Can you work these out from the model? Positions are in its coordinate system, mm. A direction names the side the tool comes from. Coordinates: 2 decimals unless noted, no trailing zeros. Loops run counter-clockwise (first coordinate to the right, second up) from the corner with the lowest first, then second, coordinate; pieces in that order, holes last. Notation, with made-up numbers: (-16.75, -31.5) -> (33.25, -31.5) arc R24 cw to (33.25, -9.5) -> close; hole circle Ø1 at (74.5, 89). An arc over 180 degrees is marked (long way). Put each result on its own line as item: value. Start each with the question number.
Item 1: We'd pull the mould along Y, two halves only. Please class faces 5 (the cylindrical face through (0.621, 21.497, 10.749)), 6 (the cylindrical face through (-5.15, 2.02, 18.59)), 7 (the flat face through (0, 15, 14.8)), 8 (the flat face through (0, 5, 3)): pulls with the +Y half, pulls with the -Y half, needs draft (parallel to the pull), parting line crosses it, or undercut.
Item 2: Will these pins go through, and if not, where does the flat tip stop? P1, Ø8, axis at y = 20.5, z = 2, coming from the +X side; P2, Ø6, axis at x = 2, z = 1, coming from the +Y side; P3, Ø0.6, axis at x = -0.5, y = -1.5, coming from the +Z side; P4, Ø6, axis at x = -2.5, z = 12, coming from the -Y side.
Item 3: If we section it at B-B on z = 13: Please give me the cut outline in (x, y), plus the area to 3 significant figures.
Item 4: For faces 1 (the flat face through (-1, -1, 3)), 2 (the flat face through (4.15, 12, 11)), 3 (the flat face through (0, -1, 2)), 4 (the cylindrical face through (5.15, 1.98, 18.59)), which set-ups out of +Z, -Z, +X, -X, +Y, -Y let a thin tool reach every point of the face, with its end or its side?
Item 5: If we section it at A-A on y = 20: Please give me the cut outline in (x, z), plus the area to 3 significant figures.
Item 6: If we section it at C-C on z = 3.5: Please give me the cut outline in (x, y).
Item 7: Please list where these lines run through material, in increasing order: L1, parallel to Y at x = 0, z = 11; L2, parallel to X at y = 20, z = 10.25; L3, parallel to Z at x = -3, y = 7.75. Write a range as from..to.
Item 8: If we section it at D-D on x = 2.5: Please give me the cut outline in (y, z), plus the area to 3 significant figures.
```python
from build123d import *

# Parameters (mm, degrees)
BOSS_EXTRUDE1_DEPTH      = 4.15
BOSS_EXTRUDE1_DEPTH_BACK = 4.15
BOSS_EXTRUDE2_DEPTH      = 18.1
BOSS_EXTRUDE3_DEPTH      = 1
BOSS_EXTRUDE4_DEPTH      = 1
SKETCH7_W                = 2
SKETCH7_H                = 2
BOSS_EXTRUDE5_DEPTH      = 1
BOSS_EXTRUDE5_DEPTH_BACK = 1


with BuildPart() as part:
    # Sketch1 → Boss-Extrude1 (new body, two sides)
    with BuildSketch(Plane(origin=(0, 0, 0), x_dir=(0, 0, -1), z_dir=(1, 0, 0))) as boss_extrude1_sk:
        with BuildLine():
            Line((-18.1, 5), (-18.1, 0))
            Line((-18.1, 0), (0, 0))
            Line((0, 0), (0, 5))
            Line((0, 5), (-6.5, 5))
            ThreePointArc((-6.5, 5), (-6.712132034, 5.087867966), (-6.8, 5.3))
            Line((-6.8, 5.3), (-6.8, 24.8))
            ThreePointArc((-6.8, 24.8), (-6.858578644, 24.941421356), (-7, 25))
            Line((-7, 25), (-14.6, 25))
            ThreePointArc((-14.6, 25), (-14.741421356, 24.941421356), (-14.8, 24.8))
            Line((-14.8, 24.8), (-14.8, 5.3))
            ThreePointArc((-14.8, 5.3), (-14.887867966, 5.087867966), (-15.1, 5))
            Line((-15.1, 5), (-18.1, 5))
        make_face()
    extrude(amount=BOSS_EXTRUDE1_DEPTH)
    extrude(boss_extrude1_sk.sketch, amount=-BOSS_EXTRUDE1_DEPTH_BACK)

    # Sketch2 → Cut-Revolve1 (revolve, cut)
    with BuildSketch(Plane(origin=(0, 0, 0), x_dir=(0, 0, -1), z_dir=(1, 0, 0))):
        Polygon((-14.8, 20), (-14.8, 22), (-14.421, 21.621), (-7.179, 21.621), (-6.8, 22), (-6.8, 20), align=None)
    revolve(axis=Axis((0, 20, 6.8), (0, 0, 1)), mode=Mode.SUBTRACT)

    # Sketch3 → Cut-Revolve2 (revolve, cut)
    with BuildSketch(Plane(origin=(0, 0, 0), x_dir=(0, 0, -1), z_dir=(1, 0, 0))):
        Polygon((-14.8, 11), (-14.8, 13), (-14.421, 12.621), (-7.179, 12.621), (-6.8, 13), (-6.8, 11), align=None)
    revolve(axis=Axis((0, 11, 6.8), (0, 0, 1)), mode=Mode.SUBTRACT)

    # Sketch4 → Boss-Extrude2 (add)
    with BuildSketch(Plane.XY):
        with BuildLine():
            Line((-4.15, 0.75), (4.15, 0.75))
            ThreePointArc((4.15, 0.75), (5.4, 2), (4.15, 3.25))
            Line((4.15, 3.25), (-4.15, 3.25))
            ThreePointArc((-4.15, 3.25), (-5.4, 2), (-4.15, 0.75))
        make_face()
    extrude(amount=BOSS_EXTRUDE2_DEPTH)

    # Sketch5 → Boss-Extrude3 (add)
    with BuildSketch(Plane.XY):
        with BuildLine():
            Line((-4.15, 0.658359214), (-4.15, 0.2))
            ThreePointArc((-4.15, 0.2), (-4.091421356, 0.058578644), (-3.95, 0))
            Line((-3.95, 0), (3.95, 0))
            ThreePointArc((3.95, 0), (4.091421356, 0.058578644), (4.15, 0.2))
            Line((4.15, 0.2), (4.15, 0.658359214))
            ThreePointArc((4.15, 0.658359214), (4.22928651, 0.897404935), (4.435714286, 1.041685153))
            ThreePointArc((4.435714286, 1.041685153), (5.15, 2), (4.435714286, 2.958314847))
            ThreePointArc((4.435714286, 2.958314847), (4.22928651, 3.102595065), (4.15, 3.341640786))
            Line((4.15, 3.341640786), (4.15, 4.8))
            ThreePointArc((4.15, 4.8), (4.091421356, 4.941421356), (3.95, 5))
            Line((3.95, 5), (-3.95, 5))
            ThreePointArc((-3.95, 5), (-4.091421356, 4.941421356), (-4.15, 4.8))
            Line((-4.15, 4.8), (-4.15, 3.341640786))
            ThreePointArc((-4.15, 3.341640786), (-4.22928651, 3.102595065), (-4.435714286, 2.958314847))
            ThreePointArc((-4.435714286, 2.958314847), (-5.15, 2), (-4.435714286, 1.041685153))
            ThreePointArc((-4.435714286, 1.041685153), (-4.22928651, 0.897404935), (-4.15, 0.658359214))
        make_face()
    extrude(amount=-BOSS_EXTRUDE3_DEPTH)

    # Sketch6 → Boss-Extrude4 (add)
    with BuildSketch(Plane.XY.offset(18.1)):
        with BuildLine():
            Line((-4.15, 0.658359214), (-4.15, 0.2))
            ThreePointArc((-4.15, 0.2), (-4.091421356, 0.058578644), (-3.95, 0))
            Line((-3.95, 0), (3.95, 0))
            ThreePointArc((3.95, 0), (4.091421356, 0.058578644), (4.15, 0.2))
            Line((4.15, 0.2), (4.15, 0.658359214))
            ThreePointArc((4.15, 0.658359214), (4.22928651, 0.897404935), (4.435714286, 1.041685153))
            ThreePointArc((4.435714286, 1.041685153), (5.15, 2), (4.435714286, 2.958314847))
            ThreePointArc((4.435714286, 2.958314847), (4.22928651, 3.102595065), (4.15, 3.341640786))
            Line((4.15, 3.341640786), (4.15, 4.8))
            ThreePointArc((4.15, 4.8), (4.091421356, 4.941421356), (3.95, 5))
            Line((3.95, 5), (-3.95, 5))
            ThreePointArc((-3.95, 5), (-4.091421356, 4.941421356), (-4.15, 4.8))
            Line((-4.15, 4.8), (-4.15, 3.341640786))
            ThreePointArc((-4.15, 3.341640786), (-4.22928651, 3.102595065), (-4.435714286, 2.958314847))
            ThreePointArc((-4.435714286, 2.958314847), (-5.15, 2), (-4.435714286, 1.041685153))
            ThreePointArc((-4.435714286, 1.041685153), (-4.22928651, 0.897404935), (-4.15, 0.658359214))
        make_face()
    extrude(amount=BOSS_EXTRUDE4_DEPTH)

    # Sketch7 → Boss-Extrude5 (add, two sides)
    with BuildSketch(Plane(origin=(0, 0, 0), x_dir=(0, 0, -1), z_dir=(1, 0, 0))) as boss_extrude5_sk:
        with Locations((-3, -1)):
            Rectangle(SKETCH7_W, SKETCH7_H)
    extrude(amount=BOSS_EXTRUDE5_DEPTH)
    extrude(boss_extrude5_sk.sketch, amount=-BOSS_EXTRUDE5_DEPTH_BACK)


solid = part.part
```
Solutions:
1. face 5: undercut
1. face 6: parting line crosses it
1. face 7: needs draft
1. face 8: pulls with the +Y half
2. P1: through
2. P2: y = 5
2. P3: z = 4
2. P4: y = 0
3. outline: (-4.15, 0) -> (4.15, 0) -> (4.15, 0.75) arc R1.25 ccw to (4.15, 3.25) -> (4.15, 25) -> (-4.15, 25) -> (-4.15, 3.25) arc R1.25 ccw to (-4.15, 0.75) -> close; hole circle Ø3.24 at (0, 11); hole circle Ø3.24 at (0, 20)
3. area: 196 mm^2
4. face 1: +Z, -Z, -X, -Y
4. face 2: +Z, -Z, +X, +Y
4. face 3: -Z, +X, -X, -Y
4. face 4: +Z, +X
5. outline: (-4.15, 6.8) -> (-2, 6.8) -> (-1.62, 7.18) -> (-1.62, 14.42) -> (-2, 14.8) -> (-4.15, 14.8) -> close; (1.62, 7.18) -> (2, 6.8) -> (4.15, 6.8) -> (4.15, 14.8) -> (2, 14.8) -> (1.62, 14.42) -> close
5. area: 40.2 mm^2
6. outline: (-4.15, 0) -> (-1, 0) -> (-1, -2) -> (1, -2) -> (1, 0) -> (4.15, 0) -> (4.15, 0.75) arc R1.25 ccw to (4.15, 3.25) -> (4.15, 5) -> (-4.15, 5) -> (-4.15, 3.25) arc R1.25 ccw to (-4.15, 0.75) -> close
7. L1: 0..9.38, 12.62..18.38, 21.62..25
7. L2: -4.15..-1.62, 1.62..4.15
7. L3: 6.8..14.8
8. outline: (0, -1) -> (5, -1) -> (5, 6.5) arc R0.3 cw to (5.3, 6.8) -> (24.8, 6.8) arc R0.2 ccw to (25, 7) -> (25, 14.6) arc R0.2 ccw to (24.8, 14.8) -> (5.3, 14.8) arc R0.3 cw to (5, 15.1) -> (5, 19.1) -> (0, 19.1) -> close
8. area: 261 mm^2
